```python
from build123d import *

# Parameters (mm, degrees)
F0_R     = 5
F0_R_2   = 2.5
F1_DEPTH = 23
F2_R     = 1.15
F3_DEPTH = 7
F4_SIZE  = 2


with BuildPart() as f1:
    # F0 (on Top) → F1 (new body)
    with BuildSketch(Plane.XY):
        with Locations((-44.115018, 43.270264)):
            Circle(F0_R)
        with Locations((-44.115018, 43.270264)):
            Circle(F0_R_2, mode=Mode.SUBTRACT)
        with Locations((-44.115018, 43.270264)):
            Circle(F0_R_2)
    extrude(amount=F1_DEPTH)

    # F2 (on face) → F3 (cut)
    with BuildSketch(Plane.XY.offset(23)):
        with Locations((-44.115018, 43.270264)):
            Circle(F2_R)
    extrude(amount=-F3_DEPTH, mode=Mode.SUBTRACT)

    # F4
    f4_edges = [f1.edges().sort_by_distance(p)[0] for p in [
        (-49.115018, 43.270264, 0),
    ]]
    chamfer(f4_edges, length=F4_SIZE)


solid = f1.part
```
Can you work these out from the model? Positions are in its coordinate system, mm. A direction names the side the tool comes from. Round coordinates to 2 decimals unless told otherwise and drop trailing zeros. Order: outer loops, then holes, each group sorted by start corner. A loop starts at its lowest first (then second) coordinate and runs counter-clockwise, first axis right, second up. Notation, with made-up numbers: (21.5, -1.5) -> (42.5, -1.5) arc R19 cw to (42.5, 16.5) -> close; hole circle Ø5 at (48.5, -39). An arc over 180 degrees is marked (long way). Return JSON: item names as keys, results as strings. Group by question number.
1. Which directions (+Z, -Z, +X, -X, +Y, -Y) give clear straight access to the entire face, cutting with the end or side of a thin tool? Please do faces 1 (the face through (-44, 43, 16)), 2 (the face through (-44, 43, 0)).
2. Will these pins go through, and if not, where does the flat tip stop? pin 1 (3 mm diameter, centred on y = 46.5, z = 10.5, fed in from +X); pin 2 (2 mm diameter, centred on y = 39.5, z = 20, fed in from +X).
3. If we section it at B-B, the plane z = 3: Write out the boundary of the cut face in (x, y).
4. We'd pull the mould along Y, two halves only. Please class faces 3 (the face through (-43, 42, 23)), 4 (the face through (-45.2, 38.39, 12.35)), 5 (the face through (-43.5, 44.24, 19.55)): released by +Y, released by -Y, zero draft, split by the parting line, or undercut.
5. If we section it at A-A, the plane z = 20.75: Write out the boundary of the cut face in (x, y), then the cut area to 3 significant figures.
6. I need wall thicknesses on line 1 (X direction, y = 42.5, z = 17.5); line 2 (Z direction, x = -43.5, y = 43.25); line 3 (Y direction, x = -46.25, z = 3.75). Which ranges of each line are inside material? Lowest first, please. Write a range as [from, to].
Output values:
{
 "1": {"face 1": "+Z", "face 2": "-Z, +X, -X, +Y, -Y"},
 "2": {"pin 1": "x = -39.42", "pin 2": "x = -39.95"},
 "3": {"outline": "circle Ø10 at (-44.12, 43.27)"},
 "4": {"face 3": "zero draft", "face 4": "split by the parting line", "face 5": "undercut"},
 "5": {"outline": "circle Ø10 at (-44.12, 43.27); hole circle Ø2.3 at (-44.12, 43.27)", "area": "74.4 mm²"},
 "6": {"line 1": "[-49.06, -44.97], [-43.26, -39.17]", "line 2": "[0, 16]", "line 3": "[38.75, 47.79]"}
}
